The listing builds one solid part. Answer for the finished solid, in the listing's coordinates (mm). Face numbers are marked on the shaded views. A direction names the side the tool comes from. Coordinates: 2 decimals unless noted, no trailing zeros. Loops run counter-clockwise (first coordinate to the right, second up) from the corner with the lowest first, then second, coordinate; pieces in that order, holes last. Notation, with made-up numbers: (-18.5, 84.5) - (-0.5, 84.5) arc R19 cw to (-0.5, 116.5) - close; hole circle Ø3 at (-19.75, 23.25). An arc over 180 degrees is marked (long way). Return JSON: item names as keys, results as strings. Group by question number.
1. Each of these flat-tipped pins is pushed along its axis until it touches: P1, Ø2, axis at x = 7, y = 8.5, coming from the -Z side; P2, Ø3.5, axis at x = 0, z = 0, coming from the +Y side; P3, Ø15.5, axis at x = 0, z = -3, coming from the -Y side; P4, Ø10, axis at y = 17, z = -15, coming from the -X side. Where does it stop, or does it pass through?
2. Find the intervals of material crossed by line 1 along X through (y, z) = (14.25, 0); line 2 along Z through (x, y) = (0, 15.2); line 3 along Z through (x, y) = (0, 14.15), in increasing order.
3. Section B-B (x = -1) is taken. Write down the section's boundary in (y, z), and give its area (3 significant figures).
4. Section D-D (z = 8.5) is taken. Write down the section's boundary in (x, y), and give its area (3 significant figures).
5. Section C-C (x = -6.5) is taken. Write down the section's boundary in (y, z), and give its area (3 significant figures).
6. Section A-A (z = 0) is taken. Write down the section's boundary in (x, y).
7. Which of the six approach directions +Z, -Z, +X, -X, +Y, -Y give full straight-line access (tool end or side, diameter ignored) to the marked faces 1, 2 and 3?
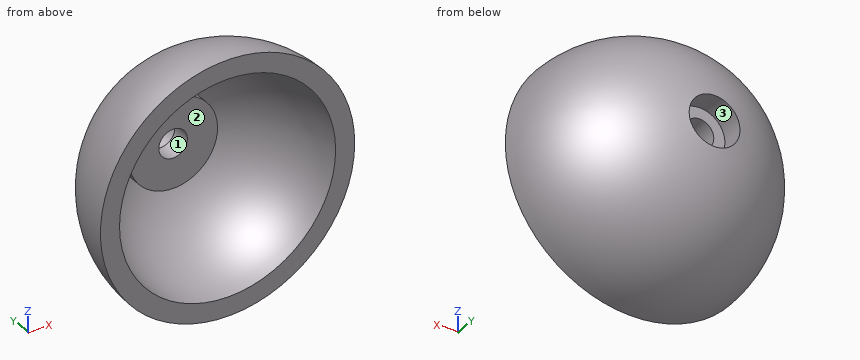
Autodesk Inventor part; units mm, degrees
ref_plane "Work Plane1" through (0, 20, 0) normal (0, 1, 0) x (-1, 0, 0)
ref_plane "YZ Plane" through (0, 0, 0) normal (1, 0, 0) x (0, 1, 0)
ref_plane "XY Plane" through (0, 0, 0) normal (0, 0, 1) x (1, 0, 0)
sketch "Sketch1" plane through (0, 0, 0) normal (0, 0, 1) x (1, 0, 0)
  line L0 (0, 0) -> (0, 20)
  line L1 (0, 0) -> (20, 0)
  arc A0 (20, 0) -> (0, 20) centre (0, 0) ccw
  line L2 (0, -4.8284) -> (0, 28.9706)
  dimension "d2" = 20
revolve "Revolution1" add sketch "Sketch1" angle 360 about axis through (0, -10, 0) along (0, 1, 0)
ref_plane "Work Plane1" through (0, 20, 0) normal (0, 1, 0) x (-1, 0, 0)
sketch "Sketch2" plane through (0, 20, 0) normal (0, 1, 0) x (-1, 0, 0)
  point P0 (0, 0)
  point P1 (0, 0)
hole "Hole1" at (0, 20, 0) direction (0, -1, 0) diameter 4.5 end through all counterbore diameter 8 counterbore depth 4
shell "Shell1" thickness 3 removed faces 1 at (13.8841, 0, 1.6858)
sketch "Sketch3" plane through (0, 0, 0) normal (0, -1, 0) x (1, 0, 0)
  circle A0 centre (0, 0) radius 5.25
  circle A1 centre (0, 0) radius 2.25
extrude "Extrusion1" cut sketch "Sketch3" against normal up to surface (13 mm away)
properties part number "Ball_Upper Half" material "Nylon 6/6"
The answers:
{
 "1": {"P1": "stops at z = -17.31", "P2": "passes through", "P3": "stops at y = 13", "P4": "stops at x = -9.37"},
 "2": {"line 1": "x = -14.03 to -9.27, -7 to -2.25, 2.25 to 7, 9.27 to 14.03", "line 2": "z = -13 to -7.61, -7 to -2.25, 2.25 to 7, 7.61 to 13", "line 3": "z = -14.13 to -9.42, -7 to -2.25, 2.25 to 7, 9.42 to 14.13"},
 "3": {"outline": "(0, -19.97) arc R19.97 ccw to (19.6, -3.87) - (16, -3.87) - (16, -2.02) - (13, -2.02) - (13, -6.93) - (15.49, -6.93) arc R16.97 cw to (0, -16.97) - close; (0, 16.97) arc R16.97 cw to (15.49, 6.93) - (13, 6.93) - (13, 2.02) - (16, 2.02) - (16, 3.87) - (19.6, 3.87) arc R19.97 ccw to (0, 19.97) - close", "area": "181 mm2"},
 "4": {"outline": "(-18.1, 0) - (-14.72, 0) arc R14.72 cw to (14.72, 0) - (18.1, 0) arc R18.1 ccw to start", "area": "174 mm2"},
 "5": {"outline": "(0, -18.91) arc R18.91 ccw to (0, 18.91) - (0, 15.71) arc R15.71 cw to (15.49, 2.6) - (13, 2.6) - (13, -2.6) - (15.49, -2.6) arc R15.71 cw to (0, -15.71) - close", "area": "188 mm2"},
 "6": {"outline": "(-20, 0) - (-17, 0) arc R17 cw to (-7, 15.49) - (-7, 13) - (-2.25, 13) - (-2.25, 16) - (-4, 16) - (-4, 19.6) arc R20 ccw to start; (2.25, 13) - (7, 13) - (7, 15.49) arc R17 cw to (17, 0) - (20, 0) arc R20 ccw to (4, 19.6) - (4, 16) - (2.25, 16) - close"},
 "7": {"face 1": "+Y, -Y", "face 2": "-Y", "face 3": "+Y"}
}
